Here's how the part is built. I have some questions about the finished solid (model axes, mm). Face numbers are marked on the shaded views. A direction names the side the tool comes from. Coordinates: 2 decimals unless noted, no trailing zeros. Write each loop counter-clockwise with the first axis right and the second up, starting at its lowest first coordinate (ties: lowest second). Pieces come first, ordered by that corner, then holes. Notation, with made-up numbers: M -25.5,70.25 L 0.5,70.25 A30 cw 0.5,92.25 Z; hole C 48.25,-16.5 d5. An arc over 180 degrees is marked long. Use one line per item in the form item = value. Start each with the question number.
1. Please list where these lines run through material, in increasing order: line 1 along X through (y, z) = (5.25, 0); line 2 along Z through (x, y) = (0, 0.75). Write a range as [from, to].
2. I want a section at A-A, the plane z = 0. List the corners of the cut face in (x, y) for me, plus the area to 3 significant figures.
3. I want a section at C-C, the plane y = 7.25. List the corners of the cut face in (x, z) for me, plus the area to 3 significant figures.
4. I'm going to push flat-ended pins straight in: pin 1 Ø1.5 at (y, z) = (1.5, -7) entering from -X; pin 2 Ø5 at (x, z) = (5.5, 5) entering from +Y; pin 3 Ø5 at (x, y) = (-3, 4) entering from +Z. Where does each tip first touch, or does it pass through?
5. I want a section at B-B, the plane x = 0. List the corners of the cut face in (y, z) for me.
6. On a 3-axis mill with a long thin cutter (end or side, diameter ignored), from which of +Z, -Z, +X, -X, +Y, -Y can I reach the whole of each face in a straight line? I mean the marked faces 1 and 2. Say none if no direction works.
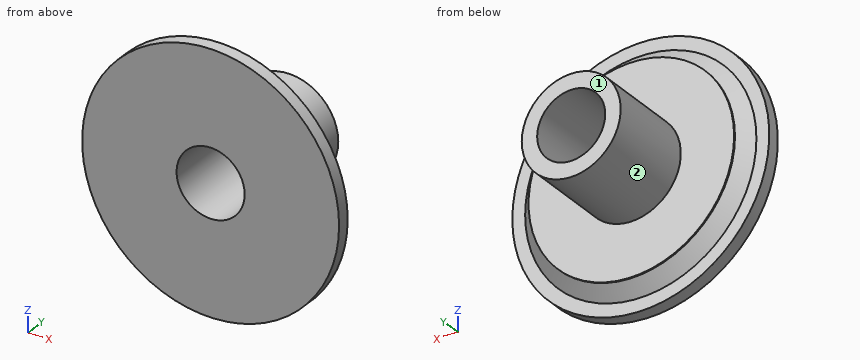
Autodesk Inventor part; units mm, degrees
ref_plane "YZ Plane" through (0, 0, 0) normal (1, 0, 0) x (0, 1, 0)
ref_plane "XZ Plane" through (0, 0, 0) normal (0, 1, 0) x (-1, 0, 0)
ref_plane "XY Plane" through (0, 0, 0) normal (0, 0, 1) x (1, 0, 0)
sketch "Boceto1" plane through (0, 0, 0) normal (0, 1, 0) x (-1, 0, 0)
  circle A0 centre (0, 0) radius 8
  dimension "d0" = 16
extrude "Extrusión1" add sketch "Boceto1" along normal blind 2.1
sketch "Boceto2" plane through (0, 2.1, 0) normal (0, 1, 0) x (1, 0, 0)
  circle A0 centre (0, 0) radius 2.65
  dimension "d3" = 5.3
extrude "Extrusión2" cut sketch "Boceto2" against normal through all
sketch "Boceto3" plane through (0, 2.1, 0) normal (0, 1, 0) x (1, 0, 0)
  circle A0 centre (0, 0) radius 3.85
  circle A1 centre (0, 0) radius 2.65
  dimension "d6" = 7.7
extrude "Extrusión3" add sketch "Boceto3" along normal blind 7
sketch "Boceto4" plane through (0, 0, 0) normal (0, -1, 0) x (1, 0, 0)
  circle A0 centre (0, 0) radius 10
  dimension "d9" = 20
extrude "Extrusión4" add sketch "Boceto4" against normal blind 1
sketch "Boceto5" plane through (0, 1, 0) normal (0, 1, 0) x (1, 0, 0)
  circle A0 centre (0, 0) radius 2.65
extrude "Extrusión5" cut sketch "Boceto5" against normal through all
chamfer "Chaflán2" distance 1 angle 45 1 edges at (8, 1, 0)
properties part number "elbowsupport"
Answer list:
q1.line_1 = [-3.85, -2.65], [2.65, 3.85]
q1.line_2 = [-10, -2.65], [2.65, 10]
q2.outline = M -10,0 L -2.65,0 L -2.65,9.1 L -3.85,9.1 L -3.85,2.1 L -8,2.1 L -8,2 L -9,1 L -10,1 Z; M 2.65,0 L 10,0 L 10,1 L 9,1 L 8,2 L 8,2.1 L 3.85,2.1 L 3.85,9.1 L 2.65,9.1 Z
q2.area = 44.3 mm²
q3.outline = C 0,0 d7.7; hole C 0,0 d5.3
q3.area = 24.5 mm²
q4.pin_1 = -7.65
q4.pin_2 = 2.1
q4.pin_3 = 8.08
q5.outline = M 0,-10 L 1,-10 L 1,-9 L 2,-8 L 2.1,-8 L 2.1,-3.85 L 9.1,-3.85 L 9.1,-2.65 L 0,-2.65 Z; M 0,2.65 L 9.1,2.65 L 9.1,3.85 L 2.1,3.85 L 2.1,8 L 2,8 L 1,9 L 1,10 L 0,10 Z
q6.face_1 = +Z, -Z, +X, -X, +Y
q6.face_2 = +Y
